```python
from build123d import *

# Parameters (mm, degrees)
SKETCH1_W                = 50
SKETCH1_H                = 50
BOSS_EXTRUDE1_DEPTH      = 5
BOSS_EXTRUDE2_DEPTH      = 5
CIRPATTERN1_COUNT        = 4
SKETCH3_R                = 10
SKETCH3_R_2              = 6
BOSS_EXTRUDE3_DEPTH      = 15
BOSS_EXTRUDE4_REACH      = 45.886
BOSS_EXTRUDE4_END_RADIUS = 10
SKETCH4_W                = 30
SKETCH4_H                = 20
SKETCH5_W                = 4
SKETCH5_H                = 4
CUT_EXTRUDE2_DEPTH       = 30


with BuildPart() as part:
    # Sketch1 → Boss-Extrude1 (new body)
    with BuildSketch(Plane(origin=(0, 0, 0), x_dir=(1, 0, 0), z_dir=(0, 1, 0))):
        Rectangle(SKETCH1_W, SKETCH1_H)
    extrude(amount=BOSS_EXTRUDE1_DEPTH)

    # Sketch2 → Boss-Extrude2 (add)
    with BuildSketch(Plane(origin=(0, 5, 0), x_dir=(1, 0, 0), z_dir=(0, 1, 0))):
        with BuildLine():
            Line((-15, 10), (-15, -10))
            ThreePointArc((-15, -10), (-17.5, -12.5), (-20, -10))
            Line((-20, -10), (-20, 10))
            ThreePointArc((-20, 10), (-17.5, 12.5), (-15, 10))
        make_face()
    boss_extrude2 = extrude(amount=BOSS_EXTRUDE2_DEPTH)

    # CirPattern1: Boss-Extrude2 ×4 about axis
    cirpattern1_axis = Axis((0, 0, 0), (0, 1, 0))
    for i in range(1, CIRPATTERN1_COUNT):
        add(boss_extrude2.rotate(cirpattern1_axis, i * 360 / CIRPATTERN1_COUNT))


with BuildPart() as body_2:
    # Sketch3 → Boss-Extrude3 (new, symmetric)
    with BuildSketch(Plane(origin=(0, 0, 0), x_dir=(0, 0, -1), z_dir=(1, 0, 0))):
        with Locations((0, -30)):
            Circle(SKETCH3_R)
        with Locations((0, -30)):
            Circle(SKETCH3_R_2, mode=Mode.SUBTRACT)
    extrude(amount=BOSS_EXTRUDE3_DEPTH, both=True)

    # Boss-Extrude4: up to this cylinder (the profile starts outside it)
    boss_extrude4_end = Plane(origin=(0, -30, 0), z_dir=(-1, 0, 0)) * Cylinder(BOSS_EXTRUDE4_END_RADIUS, 112.772, mode=Mode.PRIVATE)
    # Sketch4 → Boss-Extrude4 (add, up to the surface)
    with BuildSketch(Plane(origin=(0, -14, 0), x_dir=(-1, 0, 0), z_dir=(0, -1, 0)), mode=Mode.PRIVATE) as boss_extrude4_sk1:
        Rectangle(SKETCH4_W, SKETCH4_H)
    boss_extrude4_tool1 = extrude(boss_extrude4_sk1.sketch, amount=BOSS_EXTRUDE4_REACH, mode=Mode.PRIVATE) - boss_extrude4_end
    add(boss_extrude4_tool1.solids().sort_by_distance((0, -14, 0))[0])


    add(part.part)  # loft1 joins it to this body
    # loft from a face of the part (loft1)
    loft([body_2.faces().sort_by_distance((0, -14, 0))[0], body_2.faces().sort_by_distance((0, 0, 0))[0]])

    # Sketch5 → Cut-Extrude2 (cut)
    with BuildSketch(Plane.ZY.offset(15)):
        with Locations((0, -24)):
            Rectangle(SKETCH5_W, SKETCH5_H)
    extrude(amount=-CUT_EXTRUDE2_DEPTH, mode=Mode.SUBTRACT)


solid = body_2.part
```
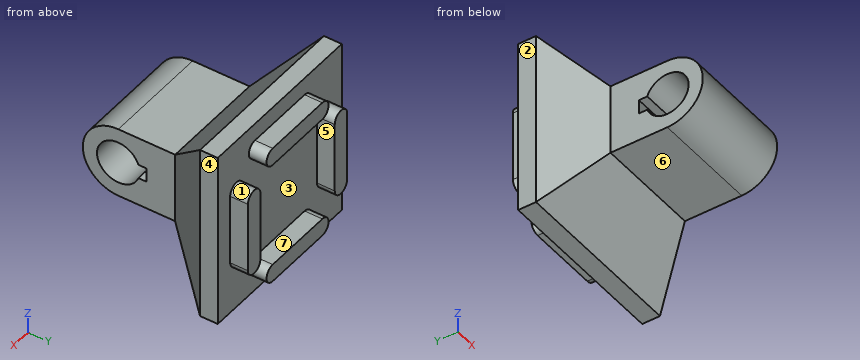
Model file for the job. Use its own axes, mm. Face numbers are marked on the shaded views. A direction names the side the tool comes from. Coordinates: 2 decimals unless noted, no trailing zeros. Loops run counter-clockwise (first coordinate to the right, second up) from the corner with the lowest first, then second, coordinate; pieces in that order, holes last. Notation, with made-up numbers: M -37.5,59 L 6.5,59 A26 ccw 6.5,76 Z; hole C -21,78 d9. An arc over 180 degrees is marked long. Use CSV: the item, a comma, the result in double quotes. Start each with the question number.
1. Probe probe 1 along Y at (x, z) = (-0.5, 0); probe 2 along Z at (x, y) = (-2.5, -30); probe 3 along X at (y, z) = (-31, -8.5). List the from-to ranges inside material, lowest first. Write a range as [from, to].
2. Flat gauge pins, fed straight in: pin 1 (2.5 mm diameter, centred on x = 1.5, y = 7, fed in from -Z); pin 2 (10 mm diameter, centred on x = 14.5, y = -25.5, fed in from -Z); pin 3 (0.7 mm diameter, centred on x = 0, y = -23.5, fed in from +Z). Where does each tip first touch, or does it go through?
3. Band-saw the part on A-A, the plane y = -23. List the corners of the cut face in (x, z).
4. Band-saw the part on B-B, the plane y = -17. List the corners of the cut face in (x, z), then the cut area to 3 significant figures.
5. Two-plate mould, pull along X, no slides. Class the marked faces 1, 2, 3 and 4: pulls with the +X half, pulls with the -X half, needs draft (parallel to the pull), parting line crosses it, or undercut.
6. Tool access for the marked faces 5, 6 and 7: list every direction of +Z, -Z, +X, -X, +Y, -Y with a clear straight run to the whole face (end or side of a thin tool).
Entries:
1,probe 1,"y = [-40, -36], [-22, 5]"
1,probe 2,"z = [-10, -6], [6, 10]"
1,probe 3,"x = [-15, 15]"
2,pin 1,"stops at z = -20"
2,pin 2,"stops at z = -10"
2,pin 3,"stops at z = 10"
3,outline,"M -15,-10 L 15,-10 L 15,-2 L -15,-2 Z; M -15,2 L 15,2 L 15,10 L -15,10 Z"
4,outline,"M -15,-10 L 15,-10 L 15,10 L -15,10 Z"
4,area,"600 mm2"
5,face 1,"undercut"
5,face 2,"pulls with the -X half"
5,face 3,"undercut"
5,face 4,"pulls with the +X half"
6,face 5,"+Z, -Z, +Y"
6,face 6,"-Z, +X, -X, -Y"
6,face 7,"+X, -X, +Y"
